CAD build for the part. Positions are in the model's coordinates, mm. A direction names the side the tool comes from. Give positions to 0.01 mm unless a question says otherwise; leave off trailing zeros. Order: outer loops, then holes, each group sorted by start corner. A loop starts at its lowest first (then second) coordinate and runs counter-clockwise, first axis right, second up. Notation, with made-up numbers: M 18,82 L 34,82 A27 ccw 34,109 Z; hole C 12.5,21.5 d5. An arc over 180 degrees is marked long. Put each result on its own line as item: value. Start each with the question number.
1) Pin check, flat tips, straight feed: pin 1 (3 mm diameter, centred on x = 12.5, y = 2.5, fed in from -Z); pin 2 (3 mm diameter, centred on y = 2.5, z = -34, fed in from -X); pin 3 (3 mm diameter, centred on x = 10, z = -41.5, fed in from -Y). Stop position of each tip, or through.
2) Drill centre lines: line 1 (Z direction, x = 11.5, y = 0.35); line 2 (Z direction, x = 11.25, y = 3.8); line 3 (X direction, y = 2.1, z = -43). Where is each one in solid material? Low to high. Write a range as [from, to].
3) Two-plate mould, pull along X, no slides. Class faces 4 (the face through (10.75, 2.32, -38.12)), 5 (the face through (11, 0, -38)), 6 (the face through (7.341, 4.854, -40.553)), 7 (the face through (14.032, 2.465, -31.488)): released by +X, released by -X, zero draft, split by the parting line, or undercut.
4) Cut at D-D (z = -39.7). Write the cut outline in (x, y), and give its area (3 significant figures).
5) Tool access for faces 1 (the face through (10.937, 4.854, -42.291)), 2 (the face through (7.562, 2.323, -40.664)), 3 (the face through (12, 5, -38)): list every direction of +Z, -Z, +X, -X, +Y, -Y with a clear straight run to the whole face (end or side of a thin tool).
6) Cut at C-C (x = 12.75). Write the cut outline in (y, z).
7) Cut at B-B (z = -34.75). Write the cut outline in (x, y).
```python
from build123d import *

# Parameters (mm, degrees)
SKETCH1_R           = 1.75
BOSS_EXTRUDE1_DEPTH = 5
CHAMFER1_SIZE       = 0.5
CHAMFER1_SIZE2      = 0.288675135


with BuildPart() as part:
    # Sketch1 → Boss-Extrude1 (new body)
    with BuildSketch(Plane(origin=(0, 0, 0), x_dir=(1, 0, 0), z_dir=(0, 1, 0))):
        with BuildLine():
            Line((15.433281573, 35.541640786), (10.961145618, 44.485912696))
            ThreePointArc((10.961145618, 44.485912696), (6.936223259, 45.827553483), (5.594582472, 41.802631123))
            Line((5.594582472, 41.802631123), (10.066718427, 32.858359214))
            ThreePointArc((10.066718427, 32.858359214), (14.091640786, 31.516718427), (15.433281573, 35.541640786))
        make_face()
        with Locations(Location((12.75, 34.2, 0), (0, 0, 270))):
            Circle(SKETCH1_R, mode=Mode.SUBTRACT)
        with BuildLine():
            Line((11.565247584, 40.482623792), (9.843111629, 43.926895702))
            ThreePointArc((9.843111629, 43.926895702), (7.495240253, 44.709519494), (6.712616461, 42.361648118))
            Line((6.712616461, 42.361648118), (8.434752416, 38.917376208))
            ThreePointArc((8.434752416, 38.917376208), (10.782623792, 38.134752416), (11.565247584, 40.482623792))
        make_face(mode=Mode.SUBTRACT)
    extrude(amount=BOSS_EXTRUDE1_DEPTH)

    # Chamfer1
    chamfer1_edges = [part.edges().sort_by_distance(p)[0] for p in [
        (10.782623792, 5, -38.134752416),
        (10.704179607, 5, -42.204759747),
        (7.495240253, 5, -44.709519494),
        (7.573684438, 5, -40.639512163),
    ]]
    chamfer1_side = [part.faces().sort_by_distance(p)[0] for p in [
        (7.993867335, 5, -37.412103611),
    ]]
    chamfer(chamfer1_edges, length=CHAMFER1_SIZE, length2=CHAMFER1_SIZE2, reference=chamfer1_side[0])


solid = part.part
```
Solution:
1. pin 1: z = -44.41
1. pin 2: x = 8.75
1. pin 3: y = 0
2. line 1: [-43.41, -40.61], [-38.8, -35.42], [-32.98, -31.47]
2. line 2: [-43.91, -41.11], [-38.48, -35.1], [-33.3, -31.6]
2. line 3: [5.28, 6.53], [10.31, 11.7]
3. face 4: undercut
3. face 5: zero draft
3. face 6: undercut
3. face 7: split by the parting line
4. outline: M 6.65,0 L 8.04,0 L 8.04,4.71 L 7.48,5 L 6.65,5 Z; M 11.75,0 L 13.35,0 L 13.35,5 L 12.25,5 L 11.75,4.71 Z
4. area: 14.9 mm²
5. face 1: +Y
5. face 2: +Y, -Y
5. face 3: +Z, -Z, +X, -X, +Y
6. outline: M 0,-40.91 L 5,-40.91 L 5,-35.95 L 0,-35.95 Z; M 0,-32.45 L 5,-32.45 L 5,-31.2 L 0,-31.2 Z
7. outline: M 9.12,0 L 11.09,0 L 11.09,5 L 9.12,5 Z; M 14.41,0 L 15.7,0 L 15.7,5 L 14.41,5 Z
